Build history of the part. All positions in model axes, mm. Give positions to 0.01 mm unless a question says otherwise; leave off trailing zeros. Write each loop counter-clockwise with the first axis right and the second up, starting at its lowest first coordinate (ties: lowest second). Pieces come first, ordered by that corner, then holes. Notation, with made-up numbers: (-24.5, 4.5) -> (-4.5, 4.5) arc R18 cw to (-4.5, 25.5) -> close; hole circle Ø9 at (43, 6). An arc over 180 degrees is marked (long way). Write item = value, one per line. Start each with the question number.
Q1. Saw through at A-A, the plane z = -53.5. List the corners of the cut face in (x, y), then the cut area to 3 significant figures.
Q2. Wall check: line 1 (Z direction, x = -98.5, y = 2.1); line 2 (X direction, y = 2.95, z = 4.5). Give the ranges that are in metal, low to high.
Q3. Drop flat-ended pins along their axis: P1, Ø0.9, axis at x = -174, y = 2, coming from the -Z side; P2, Ø0.9, axis at y = 1, z = -79, coming from the -X side; P3, Ø0.9, axis at y = 1.5, z = -79, coming from the +X side. Give the stop position or say it passes through.
from build123d import *

# Parameters (mm, degrees)
SALIENTE_EXTRUIR1_DEPTH = 3


with BuildPart() as part:
    # Croquis1 → Saliente-Extruir1 (new body)
    with BuildSketch(Plane(origin=(0, 0, 0), x_dir=(1, 0, 0), z_dir=(0, 1, 0))):
        Polygon((165, -80), (175, -80), (175, -70), (172, -70), (172, -60), (175, -60), (175, -50), (172, -50), (172, -40), (175, -40), (175, -30), (172, -30), (172, -20), (175, -20), (175, -10), (172, -10), (172, 0), (175, 0), (175, 10), (172, 10), (172, 20), (175, 20), (175, 30), (172, 30), (172, 40), (175, 40), (175, 50), (172, 50), (172, 60), (175, 60), (175, 70), (172, 70), (172, 80), (165, 80), (165, 77), (155, 77), (155, 80), (145, 80), (145, 77), (135, 77), (135, 80), (125, 80), (125, 77), (115, 77), (115, 80), (105, 80), (105, 77), (95, 77), (95, 80), (85, 80), (85, 77), (75, 77), (75, 80), (65, 80), (65, 77), (55, 77), (55, 80), (45, 80), (45, 77), (35, 77), (35, 80), (25, 80), (25, 77), (15, 77), (15, 80), (5, 80), (5, 77), (-5, 77), (-5, 80), (-15, 80), (-15, 77), (-25, 77), (-25, 80), (-35, 80), (-35, 77), (-45, 77), (-45, 80), (-55, 80), (-55, 77), (-65, 77), (-65, 80), (-75, 80), (-75, 77), (-85, 77), (-85, 80), (-95, 80), (-95, 77), (-105, 77), (-105, 80), (-115, 80), (-115, 77), (-125, 77), (-125, 80), (-135, 80), (-135, 77), (-145, 77), (-145, 80), (-155, 80), (-155, 77), (-165, 77), (-165, 80), (-172, 80), (-172, 70), (-175, 70), (-175, 60), (-172, 60), (-172, 50), (-175, 50), (-175, 40), (-172, 40), (-172, 30), (-175, 30), (-175, 20), (-172, 20), (-172, 10), (-175, 10), (-175, 0), (-172, 0), (-172, -10), (-175, -10), (-175, -20), (-172, -20), (-172, -30), (-175, -30), (-175, -40), (-172, -40), (-172, -50), (-175, -50), (-175, -60), (-172, -60), (-172, -70), (-175, -70), (-175, -80), (-165, -80), (-165, -77), (-155, -77), (-155, -80), (-145, -80), (-145, -77), (-135, -77), (-135, -80), (-125, -80), (-125, -77), (-115, -77), (-115, -80), (-105, -80), (-105, -77), (-95, -77), (-95, -80), (-85, -80), (-85, -77), (-75, -77), (-75, -80), (-65, -80), (-65, -77), (-55, -77), (-55, -80), (-45, -80), (-45, -77), (-35, -77), (-35, -80), (-25, -80), (-25, -77), (-15, -77), (-15, -80), (-5, -80), (-5, -77), (5, -77), (5, -80), (15, -80), (15, -77), (25, -77), (25, -80), (35, -80), (35, -77), (45, -77), (45, -80), (55, -80), (55, -77), (65, -77), (65, -80), (75, -80), (75, -77), (85, -77), (85, -80), (95, -80), (95, -77), (105, -77), (105, -80), (115, -80), (115, -77), (125, -77), (125, -80), (135, -80), (135, -77), (145, -77), (145, -80), (155, -80), (155, -77), (165, -77), align=None)
    extrude(amount=SALIENTE_EXTRUIR1_DEPTH)


solid = part.part
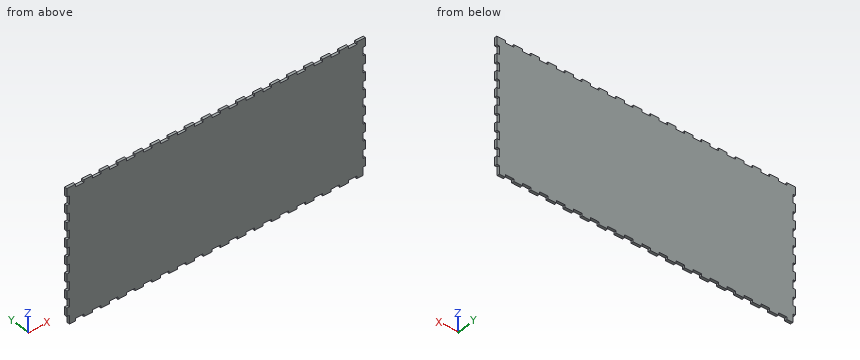
Report:
q1.outline = (-172, 0) -> (172, 0) -> (172, 3) -> (-172, 3) -> close
q1.area = 1,030 mm2
q2.line_1 = -77 to 77
q2.line_2 = -172 to 172
q3.P1 = -70
q3.P2 = -172
q3.P3 = 172
